Here's how the part is built. I have some questions about the finished solid (model axes, mm). A direction names the side the tool comes from. Round coordinates to 2 decimals unless told otherwise and drop trailing zeros. Loops run counter-clockwise (first coordinate to the right, second up) from the corner with the lowest first, then second, coordinate; pieces in that order, holes last. Notation, with made-up numbers: M 79.5,75.5 L 102.5,75.5 A17 cw 102.5,106.5 Z; hole C 24.25,41.5 d9. An arc over 180 degrees is marked long. Answer as a JSON object with one key per item and string values.
from build123d import *

# Parameters (mm, degrees)
SKETCH_1_R      = 1.85
SKETCH_1_W      = 40.374860346
SKETCH_1_H      = 10.321291022
SKETCH_1_W_2    = 7.387531562
SKETCH_1_H_2    = 3.94976935
SKETCH_1_W_3    = 20.26085389
SKETCH_1_H_3    = 4.973783626
EXTRUDE_1_DEPTH = 3


with BuildPart() as part:
    # 草图1 → 凸台-拉伸1 (new body)
    with BuildSketch(Plane(origin=(0, 0, 0), x_dir=(1, 0, 0), z_dir=(0, 1, 0))):
        with BuildLine():
            Line((49.5, -40), (-49.5, -40))
            ThreePointArc((-49.5, -40), (-50.914213562, -39.414213562), (-51.5, -38))
            Line((-51.5, -38), (-51.5, 38))
            ThreePointArc((-51.5, 38), (-50.914213562, 39.414213562), (-49.5, 40))
            Line((-49.5, 40), (49.5, 40))
            ThreePointArc((49.5, 40), (50.914213562, 39.414213562), (51.5, 38))
            Line((51.5, 38), (51.5, -38))
            ThreePointArc((51.5, -38), (50.914213562, -39.414213562), (49.5, -40))
        make_face()
        with Locations(Location((-48.296806281, 36.796806281, 0), (0, 0, 270))):
            Circle(SKETCH_1_R, mode=Mode.SUBTRACT)
        with Locations(Location((48.296806281, 36.796806281, 0), (0, 0, 270))):
            Circle(SKETCH_1_R, mode=Mode.SUBTRACT)
        with Locations(Location((48.296806281, -36.796806281, 0), (0, 0, 270))):
            Circle(SKETCH_1_R, mode=Mode.SUBTRACT)
        with Locations(Location((-48.296806281, -36.796806281, 0), (0, 0, 270))):
            Circle(SKETCH_1_R, mode=Mode.SUBTRACT)
        with Locations((0, 31.409786363)):
            Rectangle(SKETCH_1_W, SKETCH_1_H, mode=Mode.SUBTRACT)
        with Locations((37.047373629, -33.829043047)):
            Rectangle(SKETCH_1_W_2, SKETCH_1_H_2, mode=Mode.SUBTRACT)
        with Locations((0.109715815, -31.854158372)):
            Rectangle(SKETCH_1_W_3, SKETCH_1_H_3, mode=Mode.SUBTRACT)
        with Locations((-37.047373629, -33.829043047)):
            Rectangle(SKETCH_1_W_2, SKETCH_1_H_2, mode=Mode.SUBTRACT)
    extrude(amount=EXTRUDE_1_DEPTH)


solid = part.part
Item 1: I want a section at A-A, the plane x = -36. Please give me the cut outline in (y, z), then the cut area to 3 significant figures.
Resolved:
{"outline": "M 0,-40 L 3,-40 L 3,31.85 L 0,31.85 Z; M 0,35.8 L 3,35.8 L 3,40 L 0,40 Z", "area": "228 mm²"}
Item 2: I want a section at C-C, the plane y = 0.8. State how many separate pieces and enclosed holes the cut face has, then the cut area to 3 significant figures.
Resolved:
{"separate pieces": "1", "enclosed holes": "8", "area": "7,620 mm²"}
Item 3: On a 3-axis mill with a long thin cutter (end or side, diameter ignored), from which of +Z, -Z, +X, -X, +Y, -Y can I reach the whole of each face in a straight line? I mean faces 4 (the face through (-40.741, 1, 34)), 5 (the face through (-51.5, 1, 1)). Say none if no direction works.
Resolved:
{"face 4": "+Y, -Y", "face 5": "+Z, -Z, -X, +Y, -Y"}
Item 4: I want a section at B-B, the plane x = -8. Please give me the cut outline in (y, z).
Resolved:
{"outline": "M 0,-40 L 3,-40 L 3,-36.57 L 0,-36.57 Z; M 0,-26.25 L 3,-26.25 L 3,29.37 L 0,29.37 Z; M 0,34.34 L 3,34.34 L 3,40 L 0,40 Z"}
Item 5: Please list where these lines run through material, in increasing order: probe 1 along Z at (x, y) = (-6, 1.4); probe 2 along X at (y, z) = (1.2, -32); probe 3 along Z at (x, y) = (-34, 2). Write a range as from..to.
Resolved:
{"probe 1": "-40..-36.57, -26.25..29.37, 34.34..40", "probe 2": "-51.5..-20.19, 20.19..51.5", "probe 3": "-40..31.85, 35.8..40"}
Item 6: I want a section at D-D, the plane x = 17. Please give me the cut outline in (y, z), then the cut area to 3 significant figures.
Resolved:
{"outline": "M 0,-40 L 3,-40 L 3,-36.57 L 0,-36.57 Z; M 0,-26.25 L 3,-26.25 L 3,40 L 0,40 Z", "area": "209 mm²"}
Item 7: If we mould it in two halves opening along Z, with no side actions, what happens to faces 1 (the face through (0, 1, 29.367)), 2 (the face through (1, 0, -1)), 3 (the face through (50.9, 1.48, -39.43))? For each: pulls with the +Z half, pulls with the -Z half, needs draft (parallel to the pull), parting line crosses it, or undercut.
Resolved:
{"face 1": "undercut", "face 2": "needs draft", "face 3": "pulls with the -Z half"}
